Geometry check sheet. Reference: the model listing, model coordinates, mm. A direction names the side the tool comes from. Coordinates: 2 decimals unless noted, no trailing zeros. Write each loop counter-clockwise with the first axis right and the second up, starting at its lowest first coordinate (ties: lowest second). Pieces come first, ordered by that corner, then holes. Notation, with made-up numbers: M -25,43 L -8,43 A9 ccw -8,47 Z; hole C 80.25,-6.75 d8. An arc over 180 degrees is marked long. Write each question's results on one line, items separated by ' | '.
```python
from build123d import *

# Parameters (mm, degrees)
BOSS_EXTRUDE1_DEPTH = 100
SKETCH3_R           = 5
CUT_EXTRUDE2_DEPTH  = 15
BOSS_EXTRUDE5_DEPTH = 50
BOSS_EXTRUDE6_DEPTH = 48
FILLET1_R           = 1.8
SKETCH11_R          = 2.6
CUT_EXTRUDE3_DEPTH  = 15
SKETCH12_R          = 2.6
CUT_EXTRUDE4_DEPTH  = 15


with BuildPart() as part:
    # Sketch1 → Boss-Extrude1 (new body, symmetric)
    with BuildSketch(Plane.XY):
        Polygon((50, 0), (-50, 0), (-73.094010768, 40), (73.094010768, 40), align=None)
    extrude(amount=BOSS_EXTRUDE1_DEPTH, both=True)

    # Sketch3 → Cut-Extrude2 (cut)
    with BuildSketch(Plane.XZ):
        with Locations((0, 70)):
            Circle(SKETCH3_R)
        with Locations((0, -70)):
            Circle(SKETCH3_R)
        Circle(SKETCH3_R)
    extrude(amount=-CUT_EXTRUDE2_DEPTH, mode=Mode.SUBTRACT)

    # Sketch9 → Boss-Extrude5 (add)
    with BuildSketch(Plane(origin=(0, 0, -100), x_dir=(-1, 0, 0), z_dir=(0, 0, -1))):
        Polygon((50, 0), (-50, 0), (-73.094010768, 40), (73.094010768, 40), align=None)
    extrude(amount=BOSS_EXTRUDE5_DEPTH)

    # Sketch10 → Boss-Extrude6 (add)
    with BuildSketch(Plane.XY.offset(100)):
        Polygon((-50, 0), (50, 0), (73.094010768, 40), (-73.094010768, 40), align=None)
    extrude(amount=BOSS_EXTRUDE6_DEPTH)

    # Fillet1
    fillet1_edges = [part.edges().sort_by_distance(p)[0] for p in [
        (0, 0, 148),
    ]]
    fillet(fillet1_edges, radius=FILLET1_R)

    # Sketch11 → Cut-Extrude3 (cut)
    with BuildSketch(Plane.XY.offset(148)):
        with Locations((-35, 25)):
            Circle(SKETCH11_R)
        with Locations((35, 25)):
            Circle(SKETCH11_R)
    extrude(amount=-CUT_EXTRUDE3_DEPTH, mode=Mode.SUBTRACT)

    # Sketch12 → Cut-Extrude4 (cut)
    with BuildSketch(Plane(origin=(0, 0, -150), x_dir=(-1, 0, 0), z_dir=(0, 0, -1))):
        with Locations((-35, 25)):
            Circle(SKETCH12_R)
        with Locations((35, 25)):
            Circle(SKETCH12_R)
    extrude(amount=-CUT_EXTRUDE4_DEPTH, mode=Mode.SUBTRACT)


solid = part.part
```
Q1. Depth check by flat-ended pin: P1, Ø2.5, axis at x = -34.5, y = 25.5, coming from the +Z side; P2, Ø4.5, axis at x = -35, y = 25, coming from the -Z side; P3, Ø8, axis at y = 17, z = -10.5, coming from the -X side. Enter the tip coordinate at first touch or a pass-through.
Geometry check:
P1: stops at z = 133 | P2: stops at z = -135 | P3: stops at x = -62.12
Q2. Scan lines: probe 1 along Z at (x, y) = (0, 3); probe 2 along Y at (x, z) = (-35, -144.25); probe 3 along Y at (x, z) = (-34, 133.5). Record each from-to range of solid material in increasing order.
Geometry check:
probe 1: z = -150 to -75, -65 to -5, 5 to 65, 75 to 148 | probe 2: y = 0 to 22.4, 27.6 to 40 | probe 3: y = 0 to 22.6, 27.4 to 40
Q3. Sectioned sample at D-D on z = 47.5. Record the cut outline in (x, y), and give its area (3 significant figures).
Geometry check:
outline: M -73.09,40 L -50,0 L 50,0 L 73.09,40 Z | area: 4,920 mm2
Q4. Mould release check, pull along Y, two halves, no side actions. Record for faces 1 (the flat face through (-1, 20, -150)), 2 (the flat face through (-12, 0, -4)), 3 (the cylindrical face through (-34.662, 27.578, -142.605)): pulls with the +Y half, pulls with the -Y half, needs draft (parallel to the pull), parting line crosses it, or undercut.
Geometry check:
face 1: needs draft | face 2: pulls with the -Y half | face 3: undercut
Q5. Sectioned sample at C-C on x = 0. Record the cut outline in (y, z), and give its area (3 significant figures).
Geometry check:
outline: M 0,-150 L 40,-150 L 40,148 L 1.8,148 A1.8 ccw 0,146.2 L 0,75 L 15,75 L 15,65 L 0,65 L 0,5 L 15,5 L 15,-5 L 0,-5 L 0,-65 L 15,-65 L 15,-75 L 0,-75 Z | area: 11,500 mm2
Q6. Sectioned sample at B-B on y = 8. Record the cut outline in (x, z).
Geometry check:
outline: M -54.62,-150 L 54.62,-150 L 54.62,148 L -54.62,148 Z; hole C 0,-70 d10; hole C 0,0 d10; hole C 0,70 d10
Q7. Access from +Z, -Z, +X, -X, +Y, -Y to the whole of each face (thin tool, end or side, straight path). Record for faces 4 (the flat face through (-35, 25, 133)), 5 (the cylindrical face through (-1.08, 7.4, -4.88)), 6 (the flat face through (61.385, 19.72, -3.086)), 7 (the flat face through (35, 25, -135)).
Geometry check:
face 4: +Z | face 5: -Y | face 6: +Z, -Z, +X, -Y | face 7: -Z
Q8. Sectioned sample at A-A on z = -70. Record the cut outline in (x, y), and give its area (3 significant figures).
Geometry check:
outline: M -73.09,40 L -50,0 L -5,0 L -5,15 L 5,15 L 5,0 L 50,0 L 73.09,40 Z | area: 4,770 mm2
